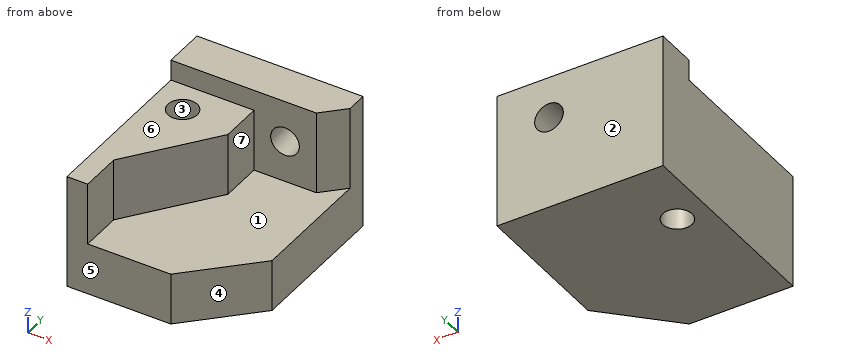
Autodesk Fusion 360 part; units mm, degrees
sketch "Sketch1" plane through (0, 0, 0) normal (0, 0, 1) x (1, 0, 0)
  line L0 (8, 10) -> (-8, 10)
  line L1 (-8, 10) -> (-8, -10)
  line L2 (-8, -10) -> (8, -10)
  line L3 (8, -10) -> (8, 10)
  line L4 (8, 10) -> (-8, -10) construction
  line L5 (-8, 10) -> (8, -10) construction
  dimension "d1" = 16
  dimension "d2" = 20
extrude "Extrude1" add sketch "Sketch1" along normal blind 13
sketch "Sketch2" plane through (8, 0, 0) normal (1, 0, 0) x (0, 1, 0)
  line L0 (-10, 0) -> (10, 0)
  line L1 (10, 0) -> (10, 13)
  line L2 (10, 13) -> (-10, 13)
  line L3 (-10, 13) -> (-10, 0)
sketch "Sketch3" plane through (0, 10, 0) normal (0, 1, 0) x (-1, 0, 0)
  line L0 (-8, 0) -> (8, 0)
  line L1 (8, 0) -> (8, 13)
  line L2 (8, 13) -> (-8, 13)
  line L3 (-8, 13) -> (-8, 0)
sketch "Sketch4" plane through (0, 0, 13) normal (0, 0, 1) x (-1, 0, 0)
  line L0 (-8, 10) -> (-8, -10)
  line L1 (-8, -10) -> (8, -10)
  line L2 (8, -10) -> (8, 10)
  line L3 (8, 10) -> (-8, 10)
  line L4 (8, -6) -> (-8, -6)
  line L5 (-8, -6) -> (-8, 10)
  line L6 (-8, 10) -> (8, 10)
  line L7 (8, 10) -> (8, -6)
  line L8 (8, -6) -> (-8, 10) construction
  line L9 (-8, -6) -> (8, 10) construction
  point P0 (0, 2)
  dimension "d5" = 16
  dimension "d6" = 16
extrude "Extrude2" cut sketch "Sketch4" against normal blind 2 contours L0 L2 L3 L4 L5 L6 L7
sketch "Sketch5" plane through (0, 0, 11) normal (0, 0, 1) x (-1, 0, 0)
  line L0 (8, 10) -> (-8, 10)
  line L1 (-8, 10) -> (-8, -6)
  line L2 (-8, -6) -> (8, -6)
  line L3 (8, -6) -> (8, 10)
  line L4 (0, -6) -> (-8, -6)
  line L5 (-8, -6) -> (-8, 10)
  line L6 (-8, 10) -> (0, 10)
  line L7 (0, 10) -> (0, -6)
  line L8 (0, -6) -> (-8, 10) construction
  line L9 (-8, -6) -> (0, 10) construction
  point P0 (-4, 2)
  dimension "d9" = 8
  dimension "d10" = 16
extrude "Extrude3" cut sketch "Sketch5" against normal blind 6 contours L0 L1 L2 L4 L5 L6 L7
sketch "Sketch6" plane through (0, 0, 11) normal (0, 0, 1) x (-1, 0, 0)
  line L0 (0, 10) -> (0, -6)
  line L1 (0, -6) -> (8, -6)
  line L2 (8, -6) -> (8, 10)
  line L3 (8, 10) -> (0, 10)
  line L4 (6, 6) -> (0, 6)
  line L5 (0, 6) -> (0, 10)
  line L6 (0, 10) -> (6, 10)
  line L7 (6, 10) -> (6, 6)
  line L8 (6, 6) -> (0, 10) construction
  line L9 (0, 6) -> (6, 10) construction
  point P0 (3, 8)
  dimension "d13" = 6
  dimension "d14" = 4
extrude "Extrude4" cut sketch "Sketch6" against normal blind 6 contours L0 L3 L4 L5 L6 L7
sketch "Sketch7" plane through (0, 0, 11) normal (0, 0, 1) x (-1, 0, 0)
  line L0 (6, 6) -> (0, 6)
  line L1 (0, 6) -> (0, -6)
  line L2 (0, -6) -> (8, -6)
  line L3 (8, -6) -> (8, 10)
  line L4 (8, 10) -> (6, 10)
  line L5 (6, 10) -> (6, 6)
  line L6 (6, 6) -> (0, -1.9864)
  line L7 (0, 6) -> (0, -1.9864)
extrude "Extrude5" cut sketch "Sketch7" against normal blind 6 contours L0 L1 L6 L7
sketch "Sketch8" plane through (0, 0, 13) normal (0, 0, 1) x (-1, 0, 0)
  line L0 (8, -6) -> (-8, -6)
  line L1 (-8, -6) -> (-8, -10)
  line L2 (-8, -10) -> (8, -10)
  line L3 (8, -10) -> (8, -6)
sketch "Sketch9" plane through (0, 0, 13) normal (0, 0, 1) x (1, 0, 0)
  line L0 (6, 6) -> (8, 8)
  line L1 (8, 8) -> (8, 6)
  line L2 (8, 6) -> (6, 6)
extrude "Extrude6" cut sketch "Sketch9" against normal blind 8
chamfer "Chamfer1" distance 6 angle 45 1 edges at (8, -10, 2.5)
sketch "Sketch10" plane through (0, 6, 0) normal (0, -1, 0) x (1, 0, 0)
  line L0 (6, 5) -> (6, 13)
  line L1 (6, 13) -> (-8, 13)
  line L2 (-8, 13) -> (-8, 11)
  line L3 (-8, 11) -> (0, 11)
  line L4 (0, 11) -> (0, 5)
  line L5 (0, 5) -> (6, 5)
  circle A0 centre (2.9897, 9) radius 1.3799
extrude "Extrude7" cut sketch "Sketch10" against normal blind 4 contours A0
sketch "Sketch11" plane through (0, 0, 11) normal (0, 0, 1) x (-1, 0, 0)
  line L0 (6, 6) -> (0, -1.9864)
  line L1 (0, -1.9864) -> (0, -6)
  line L2 (0, -6) -> (8, -6)
  line L3 (8, -6) -> (8, 10)
  line L4 (8, 10) -> (6, 10)
  line L5 (6, 10) -> (6, 6)
  circle A0 centre (5, -3) radius 1.4142
extrude "Extrude8" cut sketch "Sketch11" against normal blind 11 contours A0
Read the model definition and answer for the solid it produces. Units are mm, in the model's axes. Face numbers are marked on the shaded views. A direction names the side the tool comes from. Give positions to 0.01 mm unless a question says otherwise; leave off trailing zeros. Loops run counter-clockwise (first coordinate to the right, second up) from the corner with the lowest first, then second, coordinate; pieces in that order, holes last. Notation, with made-up numbers: (-5, -15.75) -> (22, -15.75) arc R27 cw to (22, 2.25) -> close; hole circle Ø10 at (-35.75, -30.5). An arc over 180 degrees is marked (long way). Use a Markdown table: item, result.
Q1. Section D-D, the plane x = -5 is taken. Determine the outline of the cut face in (y, z).
Solved:
| item | result |
|---|---|
| outline | (-10, 0) -> (1.59, 0) -> (1.59, 11) -> (-4.67, 11) -> (-4.67, 5) -> (-10, 5) -> close; (4.41, 0) -> (10, 0) -> (10, 13) -> (6, 13) -> (6, 11) -> (4.41, 11) -> close |
Q2. Section B-B, the plane z = 9 is taken. Determine the outline of the cut face in (x, y).
Solved:
| item | result |
|---|---|
| outline | (-8, -10) -> (-6, -10) -> (-6, -6) -> (0, 1.99) -> (0, 6) -> (1.61, 6) -> (1.61, 10) -> (-8, 10) -> close; (4.37, 6) -> (6, 6) -> (8, 8) -> (8, 10) -> (4.37, 10) -> close; hole circle Ø2.83 at (-5, 3) |
Q3. A tool of negligible diameter and unlimited length cuts with its end or side. For the marked faces 5, 6 and 7, from which of +Z, -Z, +X, -X, +Y, -Y can it reach the whole face along a straight path? Write none if from no direction.
Solved:
| item | result |
|---|---|
| face 5 | +Z, -Z, +X, -X, -Y |
| face 6 | +Z, +X, -X, -Y |
| face 7 | +Z, +X, -Y |
Q4. Determine the mould class of the marked faces 1, 2, 3 and 4 for opening direction Y: pulls with the +Y half, pulls with the -Y half, needs draft (parallel to the pull), parting line crosses it, or undercut.
Solved:
| item | result |
|---|---|
| face 1 | needs draft |
| face 2 | pulls with the +Y half |
| face 3 | undercut |
| face 4 | pulls with the -Y half |
Q5. Find the intervals of material crossed by line 1 along Y through (x, z) = (-5, 2.5); line 2 along Y through (x, z) = (-2.5, 11.75); line 3 along Z through (x, y) = (3.25, 3.5), in increasing order.
Solved:
| item | result |
|---|---|
| line 1 | y = -10 to 1.59, 4.41 to 10 |
| line 2 | y = 6 to 10 |
| line 3 | z = 0 to 5 |
Q6. Section A-A, the plane z = 6 is taken. Determine the outline of the cut face in (x, y).
Solved:
| item | result |
|---|---|
| outline | (-8, -10) -> (-6, -10) -> (-6, -6) -> (0, 1.99) -> (0, 6) -> (6, 6) -> (8, 8) -> (8, 10) -> (-8, 10) -> close; hole circle Ø2.83 at (-5, 3) |
Q7. Section C-C, the plane y = 3 is taken. Determine the outline of the cut face in (x, z), then the cut area to 3 significant figures.
Solved:
| item | result |
|---|---|
| outline | (-8, 0) -> (-6.41, 0) -> (-6.41, 11) -> (-8, 11) -> close; (-3.59, 0) -> (8, 0) -> (8, 5) -> (0, 5) -> (0, 11) -> (-3.59, 11) -> close |
| area | 96.9 mm^2 |
Q8. Each of these flat-tipped pins is pushed along its axis until it touches: pin 1 (5 mm diameter, centred on x = 6, z = 11, fed in from -Y); pin 2 (2.5 mm diameter, centred on x = -4, y = -4.5, fed in from +Z); pin 3 (1.2 mm diameter, centred on y = 3.5, z = 7.5, fed in from +X); pin 4 (2.5 mm diameter, centred on x = -5, y = 3, fed in from +Z). Where does it stop, or does it pass through?
Solved:
| item | result |
|---|---|
| pin 1 | stops at y = 6 |
| pin 2 | stops at z = 11 |
| pin 3 | stops at x = 0 |
| pin 4 | passes through |
